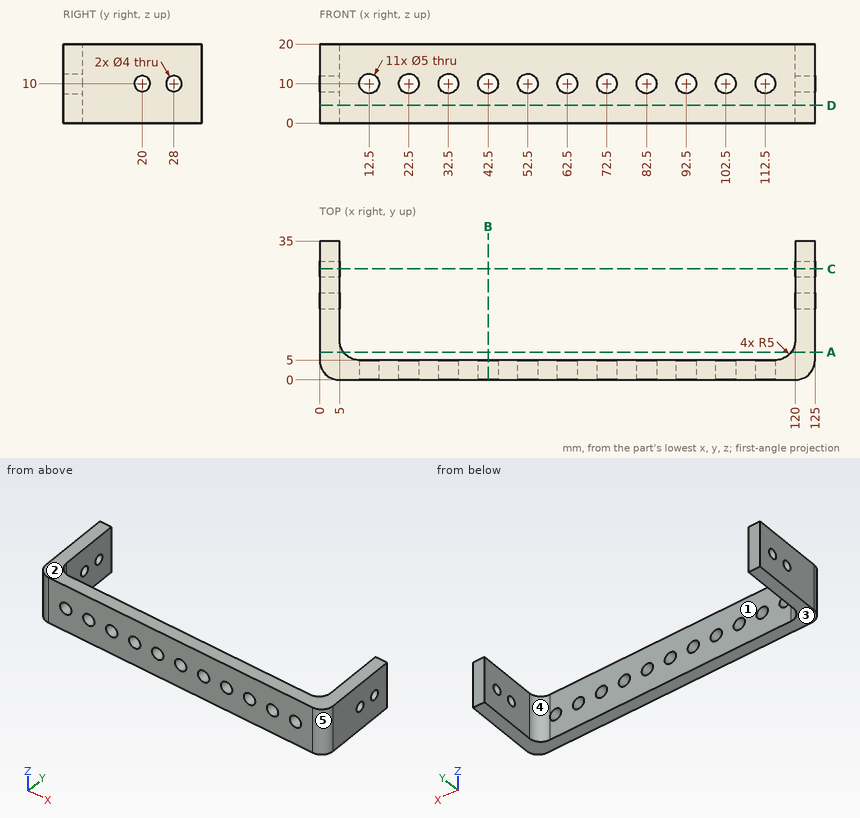
Geometry check sheet. Reference: drawing and pictorial views, mm from the part's lowest x, y, z. A direction names the side the tool comes from. Give positions to 0.01 mm unless a question says otherwise; leave off trailing zeros. Write each loop counter-clockwise with the first axis right and the second up, starting at its lowest first coordinate (ties: lowest second). Pieces come first, ordered by that corner, then holes. Notation, with made-up numbers: (-20.75, 62.25) - (13.25, 62.25) arc R22 cw to (13.25, 95.25) - close; hole circle Ø9 at (49, 9.25). An arc over 180 degrees is marked (long way). Use a Markdown table: item, result.
Q1. Section check C-C, the plane y = 28. Enter the section's corners in (x, z), then the cut area to 3 significant figures.
Computed:
| item | result |
|---|---|
| outline | (0, 0) - (5, 0) - (5, 8) - (0, 8) - close; (0, 12) - (5, 12) - (5, 20) - (0, 20) - close; (120, 0) - (125, 0) - (125, 8) - (120, 8) - close; (120, 12) - (125, 12) - (125, 20) - (120, 20) - close |
| area | 160 mm² |
Q2. Section check B-B, the plane x = 42.5. Enter the section's corners in (y, z), then the cut area to 3 significant figures.
Computed:
| item | result |
|---|---|
| outline | (0, 0) - (5, 0) - (5, 7.5) - (0, 7.5) - close; (0, 12.5) - (5, 12.5) - (5, 20) - (0, 20) - close |
| area | 75.0 mm² |
Q3. Thickness scan on L1, parallel to X at y = 14, z = 11.75; L2, parallel to Z at x = 82.5, y = 3.75; L3, parallel to Y at x = 46.5, z = 4. Record the ranges inside material, lowest first. Write a range as [from, to].
Computed:
| item | result |
|---|---|
| L1 | x = [0, 5], [120, 125] |
| L2 | z = [0, 7.5], [12.5, 20] |
| L3 | y = [0, 5] |
Q4. Go/stop test with a flat-tipped pin: P1, Ø4, axis at x = 18.5, z = 17, coming from the +Y side. Record where the tip stops, or that it passes through.
Computed:
| item | result |
|---|---|
| P1 | stops at y = 5 |
Q5. Set-up check for the marked faces 1 and 2: record each of +Z, -Z, +X, -X, +Y, -Y from which the full face is reachable in a straight line by a thin tool's end or side.
Computed:
| item | result |
|---|---|
| face 1 | +Z, -Z, +Y |
| face 2 | +Z, +X, -X, +Y, -Y |
Q6. Draft check along X on the marked faces 3, 4 and 5. Enter one of: pulls with the +X half, pulls with the -X half, needs draft (parallel to the pull), parting line crosses it, or undercut.
Computed:
| item | result |
|---|---|
| face 3 | needs draft |
| face 4 | undercut |
| face 5 | pulls with the +X half |
Q7. Section check A-A, the plane y = 7. Enter the section's corners in (x, z).
Computed:
| item | result |
|---|---|
| outline | (0, 0) - (6, 0) - (6, 20) - (0, 20) - close; (119, 0) - (125, 0) - (125, 20) - (119, 20) - close |
Q8. Section check D-D, the plane z = 4.5. Enter the section's corners in (x, y), then the cut area to 3 significant figures.
Computed:
| item | result |
|---|---|
| outline | (0, 5) arc R5 ccw to (5, 0) - (120, 0) arc R5 ccw to (125, 5) - (125, 35) - (120, 35) - (120, 10) arc R5 cw to (115, 5) - (10, 5) arc R5 cw to (5, 10) - (5, 35) - (0, 35) - close |
| area | 925 mm² |
